Geometry: final body of the model. Coordinates: model frame, mm. A direction names the side the tool comes from. Give positions to 0.01 mm unless a question says otherwise; leave off trailing zeros. Write each loop counter-clockwise with the first axis right and the second up, starting at its lowest first coordinate (ties: lowest second). Pieces come first, ordered by that corner, then holes. Notation, with made-up numbers: (48, 2) - (79, 2) arc R25 cw to (79, 14) - close; hole circle Ø7 at (50.5, 84). An arc over 180 degrees is marked (long way). Return JSON: item names as keys, results as strings.
from build123d import *

# Parameters (mm, degrees)
F0_W     = 12.7
F0_H     = 101.6
F1_DEPTH = 6.35
F2_W     = 5.08
F2_H     = 101.6
F3_DEPTH = 7.62
F4_W     = 2.54
F4_H     = 6.35
F5_DEPTH = 12.7
F7_D     = 2.54
F7_DEPTH = 12.7
F7_TIP   = 0.7630929862


with BuildPart() as f1:
    # F0 (on Top) → F1 (new body)
    with BuildSketch(Plane.XY):
        with Locations((-0.7137963548, 38.543052576)):
            Rectangle(F0_W, F0_H)
    extrude(amount=F1_DEPTH)

    # F2 (on face) → F3 (join)
    with BuildSketch(Plane.XY.offset(6.35)):
        with Locations((-4.5237963548, 38.543052576)):
            Rectangle(F2_W, F2_H)
        with Locations((3.0962036452, 38.543052576)):
            Rectangle(F2_W, F2_H)
    extrude(amount=F3_DEPTH)

    # F4 (on face) → F5 (join)
    with BuildSketch(Plane.XZ.offset(12.256947424)):
        with Locations((-0.7137963548, 3.175)):
            Rectangle(F4_W, F4_H)
    extrude(amount=F5_DEPTH)

    # F7
    with Locations(Plane(origin=(0, 89.343052576, 0), x_dir=(-1, 0, 0), z_dir=(0, 1, 0))):
        with Locations((0.7137963548, 3.175)):
            Hole(F7_D / 2, depth=F7_DEPTH)
            with Locations((0, 0, -(F7_DEPTH + F7_TIP / 2))):  # 118° drill point
                Cone(0, F7_D / 2, F7_TIP, mode=Mode.SUBTRACT)


solid = f1.part
Q1. Material intervals for probe 1 along X at (y, z) = (70.5, 10.5); probe 2 along Z at (x, y) = (-1, 4.5), sorted ascending. Write a range as [from, to].
Answer key:
{"probe 1": "x = [-7.06, -1.98], [0.56, 5.64]", "probe 2": "z = [0, 6.35]"}
Q2. Set-up query: faces 4 (the cylindrical face through (-0.879, 82.904, 4.434)), 5 (the flat face through (-1.984, 38, 10)), 6 (the flat face through (3, -12.257, 7)), 7 (the flat face through (-5, -12.257, 7)). Return all of +Z, -Z, +X, -X, +Y, -Y with unobstructed straight access to the full face (end or side cutting, diameter ignored); none if empty.
Answer key:
{"face 4": "+Y", "face 5": "+Z, +Y, -Y", "face 6": "+Z, -Z, +X, -Y", "face 7": "+Z, -Z, -X, -Y"}
Q3. Section query A-A, the plane z = 10.5. Return the cut outline in (x, y).
Answer key:
{"outline": "(-7.06, -12.26) - (-1.98, -12.26) - (-1.98, 89.34) - (-7.06, 89.34) - close; (0.56, -12.26) - (5.64, -12.26) - (5.64, 89.34) - (0.56, 89.34) - close"}
Q4. Mould query, pull axis X, two halves, no side actions, for faces 1 (the flat face through (0.556, 38, 10)), 2 (the flat face through (-5, 39, 13.97)), 3 (the flat face through (5.636, 38, 7)). Classes: pulls with the +X half, pulls with the -X half, needs draft (parallel to the pull), parting line crosses it, or undercut.
Answer key:
{"face 1": "undercut", "face 2": "needs draft", "face 3": "pulls with the +X half"}
Q5. Section query C-C, the plane x = -3.5. Return the cut outline in (y, z).
Answer key:
{"outline": "(-12.26, 0) - (89.34, 0) - (89.34, 13.97) - (-12.26, 13.97) - close"}
Q6. Pin query (flat end, axial travel): P1, Ø3, axis at y = -17.5, z = 4, coming from the +X side; P2, Ø5.5, axis at x = 3.5, z = 7, coming from the -Y side; P3, Ø1.3, axis at x = -1, y = 58, coming from the +Z side. Return the tip coordinate at first contact, or that it passes through.
Answer key:
{"P1": "stops at x = 0.56", "P2": "stops at y = -12.26", "P3": "stops at z = 6.35"}
Q7. Section query B-B, the plane y = 61. Return the cut outline in (x, z), plus the area to 3 significant figures.
Answer key:
{"outline": "(-7.06, 0) - (5.64, 0) - (5.64, 13.97) - (0.56, 13.97) - (0.56, 6.35) - (-1.98, 6.35) - (-1.98, 13.97) - (-7.06, 13.97) - close", "area": "158 mm^2"}
